Verification items for the finished model (mm, model axes). Face numbers are marked on the shaded views. A direction names the side the tool comes from. Coordinates: 2 decimals unless noted, no trailing zeros. Order: outer loops, then holes, each group sorted by start corner. A loop starts at its lowest first (then second) coordinate and runs counter-clockwise, first axis right, second up. Notation, with made-up numbers: M 30,-28.5 L 64,-28.5 A12 ccw 64,-13.5 Z; hole C 41,-37 d6. An arc over 180 degrees is marked long. Return JSON: item names as keys, results as strings.
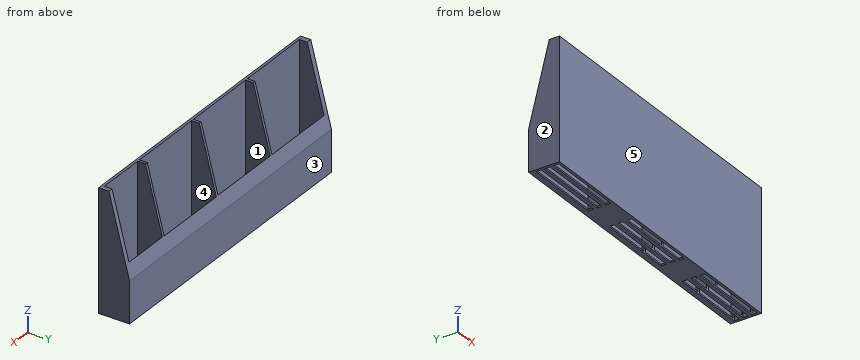
```python
from build123d import *

# Parameters (mm, degrees)
BOX_W                              = 290
BOX_H                              = 30
BOX_DEPTH                          = 117
SKETCH_W                           = 75
SKETCH_H                           = 23.820949
SKETCH_W_2                         = 48
POCKET_DEPTH                       = 115.5
POCKET001_DEPTH                    = 350
SKETCH002_W                        = 75
SKETCH002_H                        = 5
POCKET002_DEPTH                    = 5
SKETCH002_LINEARPATTERN001_2_W     = 75
SKETCH002_LINEARPATTERN001_2_H     = 5
POCKET002_LINEARPATTERN001_2_DEPTH = 5
SKETCH002_LINEARPATTERN001_3_W     = 75
SKETCH002_LINEARPATTERN001_3_H     = 5
POCKET002_LINEARPATTERN001_3_DEPTH = 5
LINEARPATTERN002_COUNT             = 3
LINEARPATTERN002_PITCH             = 8.5


with BuildPart() as part:
    # Box → Box (new body)
    with BuildSketch(Plane.XY):
        with Locations((145, 15)):
            Rectangle(BOX_W, BOX_H)
    extrude(amount=BOX_DEPTH)

    # Sketch (on Face6 of BaseFeature) → Pocket (cut)
    with BuildSketch(Plane.XY.offset(117)):
        with Locations((42.5, 14.410474)):
            Rectangle(SKETCH_W, SKETCH_H)
        with Locations((120, 14.410474)):
            Rectangle(SKETCH_W, SKETCH_H)
        with Locations((197.5, 14.481185)):
            Rectangle(SKETCH_W, SKETCH_H)
        with Locations((261.5, 14.410474)):
            Rectangle(SKETCH_W_2, SKETCH_H)
    extrude(amount=-POCKET_DEPTH, mode=Mode.SUBTRACT)

    # Sketch001 → Pocket001 (cut)
    with BuildSketch(Plane.YZ.offset(314)):
        Polygon((10, 117), (30, 40), (40, 120), align=None)
    extrude(amount=-POCKET001_DEPTH, mode=Mode.SUBTRACT)

    # Sketch002 (on Face5 of Pocket001) → Pocket002 (cut)
    with BuildSketch(Plane(origin=(0, 0, 0), x_dir=(1, 0, 0), z_dir=(0, 0, -1))):
        with Locations((40, -5)):
            Rectangle(SKETCH002_W, SKETCH002_H)
    pocket002 = extrude(amount=-POCKET002_DEPTH, mode=Mode.SUBTRACT)

    # Sketch002 LinearPattern001 2 → Pocket002 LinearPattern001 2 (cut)
    with BuildSketch(Plane(origin=(105, 0, 0), x_dir=(1, 0, 0), z_dir=(0, 0, -1))):
        with Locations((40, -5)):
            Rectangle(SKETCH002_LINEARPATTERN001_2_W, SKETCH002_LINEARPATTERN001_2_H)
    pocket002_linearpattern001_2 = extrude(amount=-POCKET002_LINEARPATTERN001_2_DEPTH, mode=Mode.SUBTRACT)

    # Sketch002 LinearPattern001 3 → Pocket002 LinearPattern001 3 (cut)
    with BuildSketch(Plane(origin=(210, 0, 0), x_dir=(1, 0, 0), z_dir=(0, 0, -1))):
        with Locations((40, -5)):
            Rectangle(SKETCH002_LINEARPATTERN001_3_W, SKETCH002_LINEARPATTERN001_3_H)
    pocket002_linearpattern001_3 = extrude(amount=-POCKET002_LINEARPATTERN001_3_DEPTH, mode=Mode.SUBTRACT)

    # LinearPattern002: Pocket002, Pocket002 LinearPattern001 2, Pocket002 LinearPattern001 3 ×3
    with Locations(*[(0, i * LINEARPATTERN002_PITCH, 0) for i in range(1, LINEARPATTERN002_COUNT)]):
        add(pocket002, mode=Mode.SUBTRACT)
        add(pocket002_linearpattern001_2, mode=Mode.SUBTRACT)
        add(pocket002_linearpattern001_3, mode=Mode.SUBTRACT)


solid = part.part
```
Q1. Material ranges on line 1 along X through (y, z) = (15.75, 53.5); line 2 along Y through (x, z) = (203, 34); line 3 along Z through (x, y) = (133, 18.25), recorded low to high.
Values:
{"line 1": "0 to 5, 80 to 82.5, 157.5 to 160, 235 to 237.5, 285.5 to 290", "line 2": "0 to 2.57, 26.39 to 30", "line 3": "0 to 1.5"}
Q2. Cross-section at C-C, the plane x = 266.5. Record the boundary of the cut face in (y, z), and give its area (3 significant figures).
Values:
{"outline": "M 0,0 L 2.5,0 L 2.5,117 L 0,117 Z; M 7.5,0 L 11,0 L 11,1.5 L 7.5,1.5 Z; M 16,0 L 19.5,0 L 19.5,1.5 L 16,1.5 Z; M 24.5,0 L 30,0 L 30,40 L 26.32,54.16 L 26.32,1.5 L 24.5,1.5 Z", "area": "479 mm^2"}
Q3. Tool access check on the marked faces 4 and 5. Record the directions out of +Z, -Z, +X, -X, +Y, -Y that give a thin tool (end or side, any length) a straight path to the whole face; none if there is none.
Values:
{"face 4": "+Z", "face 5": "+Z, -Z, +X, -X, -Y"}
Q4. Cross-section at B-B, the plane z = 22. Record the boundary of the cut face in (x, y).
Values:
{"outline": "M 0,0 L 290,0 L 290,30 L 0,30 Z; hole M 5,2.5 L 80,2.5 L 80,26.32 L 5,26.32 Z; hole M 82.5,2.5 L 157.5,2.5 L 157.5,26.32 L 82.5,26.32 Z; hole M 160,2.57 L 235,2.57 L 235,26.39 L 160,26.39 Z; hole M 237.5,2.5 L 285.5,2.5 L 285.5,26.32 L 237.5,26.32 Z"}
Q5. Go/stop test with flat-tipped pins: pin 1 (1 mm diameter, centred on x = 251, y = 9.5, fed in from +Z); pin 2 (1.2 mm diameter, centred on x = 4, y = 4.5, fed in from -Z); pin 3 (5 mm diameter, centred on x = 195.5, z = 104.5, fed in from +Y). Record where each tip stops, or that it passes through.
Values:
{"pin 1": "z = 1.5", "pin 2": "z = 5", "pin 3": "y = 2.57"}
Q6. Cross-section at D-D, the plane z = 62. Record the boundary of the cut face in (x, y), and give its area (3 significant figures).
Values:
{"outline": "M 0,0 L 290,0 L 290,24.29 L 285.5,24.29 L 285.5,2.5 L 237.5,2.5 L 237.5,24.29 L 235,24.29 L 235,2.57 L 160,2.57 L 160,24.29 L 157.5,24.29 L 157.5,2.5 L 82.5,2.5 L 82.5,24.29 L 80,24.29 L 80,2.5 L 5,2.5 L 5,24.29 L 0,24.29 Z", "area": "1,100 mm^2"}
Q7. Draft check along X on the marked faces 1, 2 and 3. Enter one of: pulls with the +X half, pulls with the -X half, needs draft (parallel to the pull), parting line crosses it, or undercut.
Values:
{"face 1": "undercut", "face 2": "pulls with the -X half", "face 3": "needs draft"}
Q8. Cross-section at A-A, the plane x = 223.5. Record the boundary of the cut face in (y, z), and give its area (3 significant figures).
Values:
{"outline": "M 0,0 L 2.5,0 L 2.5,5 L 2.57,5 L 2.57,117 L 0,117 Z; M 7.5,0 L 11,0 L 11,1.5 L 7.5,1.5 Z; M 16,0 L 19.5,0 L 19.5,1.5 L 16,1.5 Z; M 24.5,0 L 30,0 L 30,40 L 26.39,53.89 L 26.39,1.5 L 24.5,1.5 Z", "area": "483 mm^2"}
